The listing builds one solid part. Answer for the finished solid, in the listing's coordinates (mm). Coordinates: 2 decimals unless noted, no trailing zeros. Write each loop counter-clockwise with the first axis right and the second up, starting at its lowest first coordinate (ties: lowest second). Pieces come first, ordered by that corner, then holes.
(1) For a pull along Y with two mould halves and no side action, classify faces 1 (the cylindrical face through (-109.437, -122.122, 1.565)), 2 (the flat face through (119, 0, 3.572)) as +Y half, -Y half, draft (parallel to the pull), parting line (faces both ways), or undercut.
(2) The part is cut by section C-C on x = 2. Determine the outline of the cut face in (y, z) (3 decimals), plus the area to 3 significant figures.
(3) The part is cut by section A-A on y = -95.5. Determine the outline of the cut face in (x, z) (3 decimals), plus the area to 3 significant figures.
(4) Straight lines are drawn through the part: line 1 (Y direction, x = 24, z = 1.5); line 2 (X direction, y = 101.5, z = 1.1); line 3 (Y direction, x = -42.5, z = 1.5). For each, find the intervals that lie inside material, in ascending order.
(5) Given P1, Ø1.5, axis at x = -58.5, y = -72.5, coming from the +Z side (3 decimals); P2, Ø2, axis at x = 35.59, y = 88.67, coming from the +Z side, each flat-ended and moving along its own axis, determine where each tip first touches the part or whether it passes through.
(6) The part is cut by section B-B on z = 1.7. Give the number of separate pieces and of enclosed holes in the cut face, plus the area to 3 significant figures.
(7) The part is cut by section D-D on y = 70. Determine the outline of the cut face in (x, z) (3 decimals).
from build123d import *

# Parameters (mm, degrees)
F0_W     = 295.656
F0_H     = 508
F0_R     = 1.8288
F0_R_2   = 38.735
F0_R_3   = 43.8658
F1_DEPTH = 3.175
F2_W     = 57.8358
F2_H     = 62.3824
F3_DEPTH = 0.396875
F4_R     = 1.0922
F5_DEPTH = 3.175


# Not quite as in the source:
# - a length typed as a fraction of an inch, garbled in the dataset ("3 / 203.2 mm" for 3/8 in), is restored


with BuildPart() as f1:
    # F0 (on Top) → F1 (new body)
    with BuildSketch(Plane.XY):
        Rectangle(F0_W, F0_H)
        with Locations((-105.8926, -158.9786)):
            Circle(F0_R, mode=Mode.SUBTRACT)
        with Locations((-35.5854, -158.9786)):
            Circle(F0_R, mode=Mode.SUBTRACT)
        with Locations((-105.8926, -88.6714)):
            Circle(F0_R, mode=Mode.SUBTRACT)
        with Locations((-70.739, -123.825)):
            Circle(F0_R_2, mode=Mode.SUBTRACT)
        with Locations((-35.5854, -88.6714)):
            Circle(F0_R, mode=Mode.SUBTRACT)
        with Locations((29.39415, -165.16985)):
            Circle(F0_R, mode=Mode.SUBTRACT)
        with Locations((112.08385, -165.16985)):
            Circle(F0_R, mode=Mode.SUBTRACT)
        with Locations((29.39415, -82.48015)):
            Circle(F0_R, mode=Mode.SUBTRACT)
        with Locations((70.739, -123.825)):
            Circle(F0_R_3, mode=Mode.SUBTRACT)
        with Locations((112.08385, -82.48015)):
            Circle(F0_R, mode=Mode.SUBTRACT)
        with Locations((-112.08385, 82.48015)):
            Circle(F0_R, mode=Mode.SUBTRACT)
        with Locations((-70.739, 123.825)):
            Circle(F0_R_3, mode=Mode.SUBTRACT)
        with Locations((-29.39415, 82.48015)):
            Circle(F0_R, mode=Mode.SUBTRACT)
        with Locations((-112.08385, 165.16985)):
            Circle(F0_R, mode=Mode.SUBTRACT)
        with Locations((-29.39415, 165.16985)):
            Circle(F0_R, mode=Mode.SUBTRACT)
        with Locations((35.5854, 88.6714)):
            Circle(F0_R, mode=Mode.SUBTRACT)
        with Locations((70.739, 123.825)):
            Circle(F0_R_2, mode=Mode.SUBTRACT)
        with Locations((105.8926, 88.6714)):
            Circle(F0_R, mode=Mode.SUBTRACT)
        with Locations((35.5854, 158.9786)):
            Circle(F0_R, mode=Mode.SUBTRACT)
        with Locations((105.8926, 158.9786)):
            Circle(F0_R, mode=Mode.SUBTRACT)
    extrude(amount=F1_DEPTH)

    # F2 (on face) → F3 (join)
    with BuildSketch(Plane.XY.offset(3.175)):
        with Locations((118.9101, 0)):
            Rectangle(F2_W, F2_H)
        with Locations((-118.9101, 0)):
            Rectangle(F2_W, F2_H)
    extrude(amount=F3_DEPTH)

    # F4 (on face) → F5 (cut, through all)
    with BuildSketch(Plane.XY.offset(3.175)):
        with Locations((-24.3967, 0)):
            Circle(F4_R)
        with Locations((24.3967, 0)):
            Circle(F4_R)
        with Locations((-18.542, -105.283)):
            Circle(F4_R)
        with Locations((18.542, -105.283)):
            Circle(F4_R)
        with Locations((18.542, -142.367)):
            Circle(F4_R)
        with Locations((-18.542, -142.367)):
            Circle(F4_R)
        with Locations((-18.542, 142.367)):
            Circle(F4_R)
        with Locations((18.542, 142.367)):
            Circle(F4_R)
        with Locations((18.542, 105.283)):
            Circle(F4_R)
        with Locations((-18.542, 105.283)):
            Circle(F4_R)
        with Locations((-24.3967, 57.8612)):
            Circle(F4_R)
        with Locations((24.3967, 57.8612)):
            Circle(F4_R)
    extrude(amount=-F5_DEPTH, mode=Mode.SUBTRACT)


solid = f1.part
Model answer:
1. face 1: undercut
1. face 2: draft
2. outline: (-254, 0) - (254, 0) - (254, 3.175) - (-254, 3.175) - close
2. area: 1,610 mm2
3. outline: (-147.828, 0) - (-97.16, 0) - (-97.16, 3.175) - (-147.828, 3.175) - close; (-44.318, 0) - (37.244, 0) - (37.244, 3.175) - (-44.318, 3.175) - close; (104.234, 0) - (147.828, 0) - (147.828, 3.175) - (104.234, 3.175) - close
3. area: 558 mm2
4. line 1: y = -254 to -1.02, 1.02 to 56.84, 58.88 to 254
4. line 2: x = -147.83 to -108.5, -32.98 to 39.08, 102.39 to 147.83
4. line 3: y = -254 to -150.34, -97.31 to 90.26, 157.39 to 254
5. P1: stops at z = 3.175
5. P2: passes through
6. separate pieces: 1
6. enclosed holes: 32
6. area: 128,000 mm2
7. outline: (-147.828, 0) - (147.828, 0) - (147.828, 3.175) - (-147.828, 3.175) - close
